For this review, take the finished solid that the model builds, in its own axes (mm). Coordinates: 2 decimals unless noted, no trailing zeros. Write each loop counter-clockwise with the first axis right and the second up, starting at its lowest first coordinate (ties: lowest second). Pieces come first, ordered by that corner, then holes. Notation, with made-up numbers: (68.25, 1) - (106.25, 1) arc R33 cw to (106.25, 36) - close; hole circle Ø6 at (-12, -21). An arc over 180 degrees is marked (long way). Use one line per item in the form item = value. Start each with the question number.
1) For L1, parallel to Z at x = 228.6, y = -4; L2, parallel to X at y = -8, z = -70; L3, parallel to X at y = -11.25, z = 224.5, list the stretches that pass through material, from the lowest coordinate up. Write a range as from..to.
2) We need section A-A (z = 199.5). Give the boundary of the cut face in (x, y).
3) Insertion check: P1, Ø3, axis at x = -341, z = 263, coming from the -Y side; P2, Ø6, axis at x = -825, y = -6.5, coming from the +Z side; P3, Ø3, axis at x = -374.5, y = -5, coming from the +Z side. Each pin has a flat end and moves straight along its axis. Give the tip position at first contact, or say it passes through.
```python
from build123d import *

# Parameters (mm, degrees)
F1_DEPTH       = 12.7
F2_SIZE        = 31.75
F3_R           = 76.2
F5_D           = 4.826
F5_CBORE_D     = 10.16
F5_CBORE_DEPTH = 3.3528
F7_D           = 4.826


# Not quite as in the source:
# - a feature names something its author has since deleted; it is built from what else it names


with BuildPart() as f1:
    # F0 (on Front) → F1 (new body)
    with BuildSketch(Plane.XZ):
        Polygon((381, 139.7), (381, 281.3812), (-381, 281.3812), (-381, 139.7), (-1092.2, 139.7), (-1092.2, 0), (-1092.2, -139.7), (-400.1457989216, -139.7), (-381, -139.7), (-381, -281.3812), (381, -281.3812), (381, -139.7), (381, -69.85), (381, 0), (381, 69.85), align=None)
    extrude(amount=F1_DEPTH)

    # F2
    f2_edges = [f1.edges().sort_by_distance(p)[0] for p in [
        (-381, -6.35, -281.3812),
        (381, -6.35, -281.3812),
        (381, -6.35, 281.3812),
        (-381, -6.35, 281.3812),
        (-1092.2, -6.35, -139.7),
        (-1092.2, -6.35, 139.7),
    ]]
    chamfer(f2_edges, length=F2_SIZE)

    # F3
    f3_edges = [f1.edges().sort_by_distance(p)[0] for p in [
        (-381, -6.35, 139.7),
        (-381, -6.35, -139.7),
    ]]
    fillet(f3_edges, radius=F3_R)

    # F5 (through all)
    with Locations(Plane.XZ.offset(12.7)):
        with Locations((-340.5124, 263.9314), (-315.1124, 263.9314), (-315.1124, 221.0562), (-340.5124, 221.0562), (315.1124, 263.9314), (340.5124, 263.9314), (340.5124, 221.0562), (315.1124, 221.0562), (340.5124, -221.0562), (315.1124, -221.0562), (315.1124, -263.9314), (340.5124, -263.9314), (-315.1124, -221.0562), (-340.5124, -221.0562), (-340.5124, -263.9314), (-315.1124, -263.9314)):
            CounterBoreHole(F5_D / 2, F5_CBORE_D / 2, F5_CBORE_DEPTH)

    # F7 (through all)
    with Locations(Plane.XZ.offset(12.7)):
        with Locations((-76.2, 69.85), (228.6, 69.85), (228.6, -69.85), (-76.2, -69.85)):
            Hole(F7_D / 2)


solid = f1.part
```
Determined:
q1.L1 = -281.38..-72.26, -67.44..67.44, 72.26..281.38
q1.L2 = -1092.2..-78.61, -73.79..226.19, 231.01..381
q1.L3 = -381..-344.25, -336.78..-318.85, -311.38..311.38, 318.85..336.78, 344.25..381
q2.outline = (-382.79, -12.7) - (381, -12.7) - (381, 0) - (-382.79, 0) - close
q3.P1 = -9.35
q3.P2 = 139.7
q3.P3 = 257.63
